Input: part model. Units: mm. Frame: model coordinates. A direction names the side the tool comes from. Coordinates: 2 decimals unless noted, no trailing zeros. Order: outer loops, then holes, each group sorted by start corner. A loop starts at its lowest first (then second) coordinate and runs counter-clockwise, first axis right, second up. Notation, with made-up numbers: (5, -27) -> (10, -27) arc R21 cw to (10, 1) -> close; hole circle Ø8 at (-6, -8). An arc over 180 degrees is marked (long way). Use one line per item in the form item = value. Start each with the question number.
1) Access query for faces 4 (the cylindrical face through (-52.39, 1.43, 50.115)), 5 (the flat face through (24.71, 1, 0)), 6 (the flat face through (13, 1, -28.1)), 7 (the flat face through (-36.51, 1, 23)). Directions: +Z, -Z, +X, -X, +Y, -Y. A direction counts if a zero-diameter tool reaches every point of the face in a straight line with its end or side. Return the directions, or none.
2) Section query D-D on z = -58. Output: boundary loops of the cut face in (x, y).
3) Section query B-B on y = 1.3. Output: boundary loops of the cut face in (x, z), then the cut area to 3 significant figures.
4) Ray query, line 1 along Z through (x, y) = (-1, 1.3); line 2 along X through (y, z) = (2.4, 29); line 3 along X through (y, z) = (0.55, -2). Return the intervals inside material, ascending.
5) Draft query along Z for faces 1 (the flat face through (31, 1, 15)), 2 (the cylindrical face through (1.15, 1.43, -72.49)), 3 (the cylindrical face through (-0.565, 1.43, 44.994)). Return one class per face: pulls with the +Z half, pulls with the -Z half, needs draft (parallel to the pull), parting line crosses it, or undercut.
6) Section query A-A on z = -24.5. Output: boundary loops of the cut face in (x, y), then the cut area to 3 significant figures.
7) Pin query (flat end, axial travel): pin 1 (1.4 mm diameter, centred on x = -1, y = 2, fed in from +Z); pin 2 (1.4 mm diameter, centred on y = 1, z = 26, fed in from +X); pin 3 (1 mm diameter, centred on x = -49, y = 2, fed in from -Z). Return the tip coordinate at first contact, or that it passes through.
8) Section query C-C on x = 28. Output: boundary loops of the cut face in (y, z), then the cut area to 3 significant figures.
from build123d import *

# Parameters (mm, degrees)
BOSS_EXTRUDE1_DEPTH  = 2.9
SOLENOID_PLACEMENT_W = 37.4
SOLENOID_PLACEMENT_H = 63.8
CUT_EXTRUDE1_DEPTH   = 103.571487266
CUT_EXTRUDE3_DEPTH   = 103.571487266
SKETCH4_W            = 13
SKETCH4_H            = 26.3
CUT_EXTRUDE4_DEPTH   = 98.774792252


with BuildPart() as part:
    # Sketch1 → Boss-Extrude1 (new body)
    with BuildSketch(Plane(origin=(0, 0, 0), x_dir=(1, 0, 0), z_dir=(0, 1, 0))):
        with BuildLine():
            ThreePointArc((33.29110537, -64.404598464), (0, 72.5), (-33.29110537, -64.404598464))
            ThreePointArc((-33.29110537, -64.404598464), (0, -44.989799638), (33.29110537, -64.404598464))
        make_face()
    extrude(amount=BOSS_EXTRUDE1_DEPTH)

    # solenoid placement → Cut-Extrude1 (cut, through all)
    with BuildSketch(Plane(origin=(0, 2.9, 0), x_dir=(1, 0, 0), z_dir=(0, 1, 0))):
        with Locations((0, -3.8)):
            Rectangle(SOLENOID_PLACEMENT_W, SOLENOID_PLACEMENT_H)
    extrude(amount=-CUT_EXTRUDE1_DEPTH, mode=Mode.SUBTRACT)

    # Sketch3 → Cut-Extrude3 (cut, through all)
    with BuildSketch(Plane(origin=(0, 2.9, 0), x_dir=(1, 0, 0), z_dir=(0, 1, 0))):
        with BuildLine():
            Line((-36.51, -15), (-36.51, -31))
            Line((-36.51, -31), (-65.538156825, -31))
            ThreePointArc((-65.538156825, -31), (-72.5, 0), (-65.538156825, 31))
            Line((-65.538156825, 31), (-36.51, 31))
            Line((-36.51, 31), (-36.51, 15))
            Line((-36.51, 15), (-24.71, 15))
            Line((-24.71, 15), (-24.71, -15))
            Line((-24.71, -15), (-36.51, -15))
        make_face()
        with BuildLine():
            Line((36.51, 31), (65.538156825, 31))
            ThreePointArc((65.538156825, 31), (72.5, 0), (65.538156825, -31))
            Line((65.538156825, -31), (36.51, -31))
            Line((36.51, -31), (36.51, -15))
            Line((36.51, -15), (24.71, -15))
            Line((24.71, -15), (24.71, 15))
            Line((24.71, 15), (36.51, 15))
            Line((36.51, 15), (36.51, 31))
        make_face()
    extrude(amount=-CUT_EXTRUDE3_DEPTH, mode=Mode.SUBTRACT)

    # Sketch4 → Cut-Extrude4 (cut, through all)
    with BuildSketch(Plane(origin=(0, 2.9, 0), x_dir=(1, 0, 0), z_dir=(0, 1, 0))):
        with Locations((0, 41.25)):
            Rectangle(SKETCH4_W, SKETCH4_H)
    extrude(amount=-CUT_EXTRUDE4_DEPTH, mode=Mode.SUBTRACT)


solid = part.part
Answers below:
q1.face_4 = +Z, -X, +Y, -Y
q1.face_5 = +X, +Y, -Y
q1.face_6 = +Y, -Y
q1.face_7 = -X, +Y, -Y
q2.outline = (-43.5, 0) -> (43.5, 0) -> (43.5, 2.9) -> (-43.5, 2.9) -> close
q3.outline = (-65.54, -31) arc R72.5 ccw to (65.54, -31) -> (36.51, -31) -> (36.51, -15) -> (24.71, -15) -> (24.71, 15) -> (36.51, 15) -> (36.51, 31) -> (65.54, 31) arc R72.5 ccw to (33.29, 64.4) arc R38.25 cw to (-33.29, 64.4) arc R72.5 ccw to (-65.54, 31) -> (-36.51, 31) -> (-36.51, 15) -> (-24.71, 15) -> (-24.71, -15) -> (-36.51, -15) -> (-36.51, -31) -> close; hole (-18.7, -28.1) -> (-6.5, -28.1) -> (-6.5, -54.4) -> (6.5, -54.4) -> (6.5, -28.1) -> (18.7, -28.1) -> (18.7, 35.7) -> (-18.7, 35.7) -> close
q3.area = 7,610 mm^2
q4.line_1 = -72.49 to -54.4, 35.7 to 45
q4.line_2 = -36.51 to -18.7, 18.7 to 36.51
q4.line_3 = -24.71 to -18.7, 18.7 to 24.71
q5.face_1 = undercut
q5.face_2 = pulls with the -Z half
q5.face_3 = pulls with the +Z half
q6.outline = (-36.51, 0) -> (-18.7, 0) -> (-18.7, 2.9) -> (-36.51, 2.9) -> close; (18.7, 0) -> (36.51, 0) -> (36.51, 2.9) -> (18.7, 2.9) -> close
q6.area = 103 mm^2
q7.pin_1 = 45.03
q7.pin_2 = 36.51
q7.pin_3 = -53.89
q8.outline = (0, -66.87) -> (2.9, -66.87) -> (2.9, -15) -> (0, -15) -> close; (0, 15) -> (2.9, 15) -> (2.9, 57.18) -> (0, 57.18) -> close
q8.area = 273 mm^2
